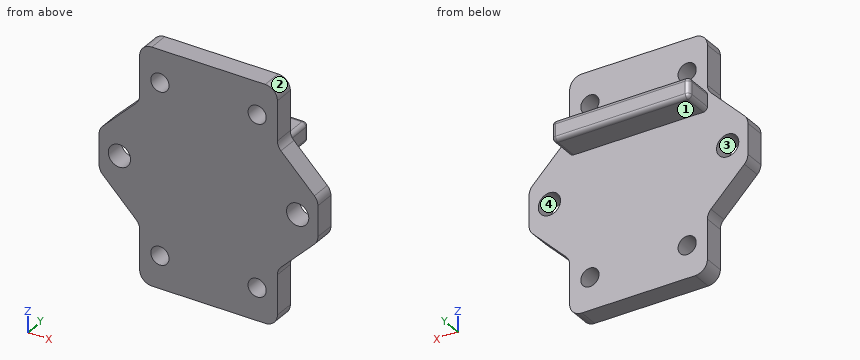
from build123d import *

# Parameters (mm, degrees)
SKETCH1_R           = 2.25
SKETCH1_R_2         = 2.75
BOSS_EXTRUDE1_DEPTH = 2.5
FILLET2_R           = 3
SKETCH2_W           = 34
SKETCH2_H           = 5
BOSS_EXTRUDE2_DEPTH = 7
FILLET3_R           = 1


with BuildPart() as part:
    # Sketch1 → Boss-Extrude1 (new, symmetric)
    with BuildSketch(Plane(origin=(0, 0, 0), x_dir=(1, 0, 0), z_dir=(0, 1, 0))):
        Polygon((-17, -29), (17, -29), (17, -15), (27, -5), (27, 5), (17, 15), (17, 29), (-17, 29), (-17, 15), (-27, 5), (-27, -5), (-17, -15), align=None)
        with Locations(Location((-12, 21, 0), (0, 0, 270))):
            Circle(SKETCH1_R, mode=Mode.SUBTRACT)
        with Locations(Location((12, 21, 0), (0, 0, 270))):
            Circle(SKETCH1_R, mode=Mode.SUBTRACT)
        with Locations(Location((-12, -21, 0), (0, 0, 270))):
            Circle(SKETCH1_R, mode=Mode.SUBTRACT)
        with Locations(Location((12, -21, 0), (0, 0, 270))):
            Circle(SKETCH1_R, mode=Mode.SUBTRACT)
        with Locations(Location((-22, 0, 0), (0, 0, 270))):
            Circle(SKETCH1_R_2, mode=Mode.SUBTRACT)
        with Locations(Location((22, 0, 0), (0, 0, 90))):
            Circle(SKETCH1_R_2, mode=Mode.SUBTRACT)
    extrude(amount=BOSS_EXTRUDE1_DEPTH, both=True)

    # Fillet2
    fillet2_edges = [part.edges().sort_by_distance(p)[0] for p in [
        (17, 0, -15),
        (27, 0, -5),
        (27, 0, 5),
        (17, 0, 15),
        (17, 0, 29),
        (-17, 0, 29),
        (-17, 0, 15),
        (-27, 0, 5),
        (-27, 0, -5),
        (-17, 0, -15),
        (-17, 0, -29),
        (17, 0, -29),
    ]]
    fillet(fillet2_edges, radius=FILLET2_R)

    # Sketch2 → Boss-Extrude2 (add)
    with BuildSketch(Plane(origin=(0, 2.5, 0), x_dir=(1, 0, 0), z_dir=(0, 1, 0))):
        with Locations((0, -12.5)):
            Rectangle(SKETCH2_W, SKETCH2_H)
    extrude(amount=BOSS_EXTRUDE2_DEPTH)

    # Fillet3
    fillet3_edges = [part.edges().sort_by_distance(p)[0] for p in [
        (-17, 6, 10),
        (-17, 6, 15),
        (17, 6, 15),
        (17, 6, 10),
        (-17, 9.5, 12.5),
        (0, 9.5, 15),
        (17, 9.5, 12.5),
        (0, 9.5, 10),
    ]]
    fillet(fillet3_edges, radius=FILLET3_R)


solid = part.part
Read the model definition and answer for the solid it produces. Units are mm, in the model's axes. Face numbers are marked on the shaded views. Round coordinates to 2 decimals unless told otherwise and drop trailing zeros. Write each loop counter-clockwise with the first axis right and the second up, starting at its lowest first coordinate (ties: lowest second). Pieces come first, ordered by that corner, then holes. Notation, with made-up numbers: (87, 11) - (141, 11) arc R13 ccw to (141, 15) - close; hole circle Ø9 at (-28.5, 62.25). An arc over 180 degrees is marked (long way). Use a Markdown table: item, result.
(1) The part is cut by section C-C (y = 7.5). Write down the section's boundary in (x, z).
Reported:
| item | result |
|---|---|
| outline | (-17, 11) arc R1 ccw to (-16, 10) - (16, 10) arc R1 ccw to (17, 11) - (17, 14) arc R1 ccw to (16, 15) - (-16, 15) arc R1 ccw to (-17, 14) - close |
(2) The part is cut by section A-A (x = -12). Write down the section's boundary in (y, z).
Reported:
| item | result |
|---|---|
| outline | (-2.5, -29) - (2.5, -29) - (2.5, -23.25) - (-2.5, -23.25) - close; (-2.5, -18.75) - (2.5, -18.75) - (2.5, 10) - (8.5, 10) arc R1 ccw to (9.5, 11) - (9.5, 14) arc R1 ccw to (8.5, 15) - (2.5, 15) - (2.5, 18.75) - (-2.5, 18.75) - close; (-2.5, 23.25) - (2.5, 23.25) - (2.5, 29) - (-2.5, 29) - close |
(3) Straight lines are drawn through the part: line 1 along X through (y, z) = (1.5, -21); line 2 along X through (y, z) = (1.2, 0); line 3 along Y through (x, z) = (23, 3.5). For each, find the intervals that lie inside material, in ascending order. Write a range as [from, to].
Reported:
| item | result |
|---|---|
| line 1 | [-17, -14.25], [-9.75, 9.75], [14.25, 17] |
| line 2 | [-27, -24.75], [-19.25, 19.25], [24.75, 27] |
| line 3 | [-2.5, 2.5] |
(4) The part is cut by section B-B (z = 0). Write down the section's boundary in (x, y), then the cut area to 3 significant figures.
Reported:
| item | result |
|---|---|
| outline | (-27, -2.5) - (-24.75, -2.5) - (-24.75, 2.5) - (-27, 2.5) - close; (-19.25, -2.5) - (19.25, -2.5) - (19.25, 2.5) - (-19.25, 2.5) - close; (24.75, -2.5) - (27, -2.5) - (27, 2.5) - (24.75, 2.5) - close |
| area | 215 mm2 |
(5) The mould has two halves that part along Z. Classify the marked faces 1, 2, 3 and 4: released by +Z, released by -Z, zero draft, split by the parting line, or undercut.
Reported:
| item | result |
|---|---|
| face 1 | released by -Z |
| face 2 | released by +Z |
| face 3 | undercut |
| face 4 | undercut |
(6) Each of these flat-tipped pins is pushed along its axis until it touches: pin 1 Ø4 at (x, y) = (19.5, 1) entering from -Z; pin 2 Ø4 at (x, z) = (12, 21) entering from -Y; pin 3 Ø0.9 at (y, z) = (5.5, 12) entering from +X; pin 4 Ø5.5 at (y, z) = (-1, -20) entering from -X. Where does it stop, or does it pass through?
Reported:
| item | result |
|---|---|
| pin 1 | z = -14.58 |
| pin 2 | through |
| pin 3 | x = 17 |
| pin 4 | x = -17 |
(7) The part is cut by section D-D (x = 1). Write down the section's boundary in (y, z), then the cut area to 3 significant figures.
Reported:
| item | result |
|---|---|
| outline | (-2.5, -29) - (2.5, -29) - (2.5, 10) - (8.5, 10) arc R1 ccw to (9.5, 11) - (9.5, 14) arc R1 ccw to (8.5, 15) - (2.5, 15) - (2.5, 29) - (-2.5, 29) - close |
| area | 325 mm2 |
